```python
from build123d import *

# Parameters (mm, degrees)
SKETCH3_R          = 1.5
SKETCH3_R_2        = 0.7
CUT_EXTRUDE1_DEPTH = 1.2


with BuildPart() as part:
    # Sketch1 → Revolve1 (revolve)
    with BuildSketch(Plane.XY):
        Polygon((4.45, 0), (4.45, 2.8), (5.45, 2.8), (5.45, 0.6), (19.2, 0.6), (19.2, 4), (20.1, 4.7), (20.1, 5.4), (21, 5.4), (21, 1), (22.4, 1), (22.4, 0), align=None)
    revolve1 = revolve(axis=Axis((0, -5.4, 0), (0, 1, 0)))

    # Mirror1: Revolve1 across plane
    add(revolve1.mirror(Plane(origin=(22.4, 0, 0), x_dir=(0, 0, 1), z_dir=(0, -1, 0))))

    # Sketch3 → Cut-Extrude1 (cut)
    with BuildSketch(Plane(origin=(0, 0.6, 0), x_dir=(1, 0, 0), z_dir=(0, 1, 0))):
        with Locations(Location((0, 10, 0), (0, 0, 180))):
            Circle(SKETCH3_R)
        with Locations(Location((-8.660254038, -5, 0), (0, 0, 180))):
            Circle(SKETCH3_R)
        with Locations(Location((8.660254038, -5, 0), (0, 0, 180))):
            Circle(SKETCH3_R)
        with Locations(Location((-7.837529904, 4.525, 0), (0, 0, 180))):
            Circle(SKETCH3_R_2)
        with Locations(Location((7.837529904, 4.525, 0), (0, 0, 180))):
            Circle(SKETCH3_R_2)
        with Locations(Location((0, -9.05, 0), (0, 0, 180))):
            Circle(SKETCH3_R_2)
    extrude(amount=-CUT_EXTRUDE1_DEPTH, mode=Mode.SUBTRACT)

    # Cut-Extrude2 cone 1 section (through the dimple's axis) → Cut-Extrude2 (revolve, cut)
    with BuildSketch(Plane(origin=(0, 0.6, 9.05), x_dir=(0, 0, 1), z_dir=(1, 0, 0))):
        Polygon((0, 0), (0.95, 0), (0, 0.95), align=None)
    revolve(axis=Axis((0, 0.6, 9.05), (0, -1, 0)), mode=Mode.SUBTRACT)

    # Cut-Extrude2 cone 2 section (through the dimple's axis) → Cut-Extrude2 cone 2 (revolve, cut)
    with BuildSketch(Plane(origin=(7.837529904, 0.6, -4.525), x_dir=(0, 0, 1), z_dir=(1, 0, 0))):
        Polygon((0, 0), (0.95, 0), (0, 0.95), align=None)
    revolve(axis=Axis((7.837529904, 0.6, -4.525), (0, -1, 0)), mode=Mode.SUBTRACT)

    # Cut-Extrude2 cone 3 section (through the dimple's axis) → Cut-Extrude2 cone 3 (revolve, cut)
    with BuildSketch(Plane(origin=(-7.837529904, 0.6, -4.525), x_dir=(0, 0, 1), z_dir=(1, 0, 0))):
        Polygon((0, 0), (0.95, 0), (0, 0.95), align=None)
    revolve(axis=Axis((-7.837529904, 0.6, -4.525), (0, -1, 0)), mode=Mode.SUBTRACT)

    # Cut-Extrude3 cone 1 section (through the dimple's axis) → Cut-Extrude3 (revolve, cut)
    with BuildSketch(Plane(origin=(7.837529904, -0.6, -4.525), x_dir=(0, 0, -1), z_dir=(1, 0, 0))):
        Polygon((0, 0), (0.95, 0), (0, 0.95), align=None)
    revolve(axis=Axis((7.837529904, -0.6, -4.525), (0, 1, 0)), mode=Mode.SUBTRACT)

    # Cut-Extrude3 cone 2 section (through the dimple's axis) → Cut-Extrude3 cone 2 (revolve, cut)
    with BuildSketch(Plane(origin=(0, -0.6, 9.05), x_dir=(0, 0, -1), z_dir=(1, 0, 0))):
        Polygon((0, 0), (0.95, 0), (0, 0.95), align=None)
    revolve(axis=Axis((0, -0.6, 9.05), (0, 1, 0)), mode=Mode.SUBTRACT)

    # Cut-Extrude3 cone 3 section (through the dimple's axis) → Cut-Extrude3 cone 3 (revolve, cut)
    with BuildSketch(Plane(origin=(-7.837529904, -0.6, -4.525), x_dir=(0, 0, -1), z_dir=(1, 0, 0))):
        Polygon((0, 0), (0.95, 0), (0, 0.95), align=None)
    revolve(axis=Axis((-7.837529904, -0.6, -4.525), (0, 1, 0)), mode=Mode.SUBTRACT)


solid = part.part
```
Could you check a few things on this model? Use its own coordinates, in mm. A direction names the side the tool comes from. Round coordinates to 2 decimals unless told otherwise and drop trailing zeros.
Q1. On a 3-axis mill with a long thin cutter (end or side, diameter ignored), from which of +Z, -Z, +X, -X, +Y, -Y can I reach the whole of each face in a straight line? I mean faces 1 (the cylindrical face through (5.198, 1.685, -1.637)), 2 (the cylindrical face through (5.198, -1.685, -1.637)), 3 (the cylindrical face through (0.325, 0.008, -11.464)). Say none if no direction works.
Q2. Thinking about a two-plate mould opening in X: for faces 4 (the cylindrical face through (-8.484, 0.005, -4.793)), 5 (the cylindrical face through (20.03, 3.17, -6.31)), 6 (the flat face through (-7, -1, -20)), 7 (the cylindrical face through (0.152, 0.005, 8.367)), which applies, pulls with the +X half, pulls with the -X half, needs draft (parallel to the pull), parting line crosses it, or undercut?
Q3. Please list where these lines run through material, in increasing order: L1, parallel to Z at x = 0, y = -0.1; L2, parallel to X at y = -1.6, z = 0; L3, parallel to Z at x = 0, y = -0.9.
Q4. For P1, Ø3, axis at y = 0, z = -17, coming from the -X side; P2, Ø6, axis at x = 3, z = 0, coming from the -Y side; P3, Ø1.5, axis at y = 2.5, z = 15, coming from the -X side; P4, Ø1.3, axis at x = -7.84, z = -4.53, coming from the -Y side, each with a flat end and sliding along its axis, tell me the tip position at first contact or that it passes through.
Answer below:
1. face 1: +Y
1. face 2: -Y
1. face 3: +Y, -Y
2. face 4: undercut
2. face 5: parting line crosses it
2. face 6: needs draft
2. face 7: undercut
3. L1: z = -22.4 to -11.5, -8.5 to -4.45, 4.45 to 8.35, 9.75 to 22.4
3. L2: x = -21 to -19.2, -5.45 to -4.45, 4.45 to 5.45, 19.2 to 21
3. L3: z = -22.4 to -19.2, -5.45 to -4.45, 4.45 to 5.45, 19.2 to 22.4
4. P1: stops at x = -16.17
4. P2: stops at y = -2.8
4. P3: stops at x = -15.43
4. P4: passes through
